For this review, take the finished solid that the model builds, in its own axes (mm). Face numbers are marked on the shaded views. A direction names the side the tool comes from. Give positions to 0.01 mm unless a question says otherwise; leave off trailing zeros. Order: outer loops, then holes, each group sorted by start corner. A loop starts at its lowest first (then second) coordinate and runs counter-clockwise, first axis right, second up. Notation, with made-up numbers: (-7.75, 88) - (12.25, 88) arc R8 cw to (12.25, 98) - close; hole circle Ø5 at (44.5, -34). An arc over 180 degrees is marked (long way). Use a Markdown table: item, result. Add a question column.
1) Wall thickness on L1, parallel to Y at x = -84, z = -15; L2, parallel to Z at x = 92, y = 3: over which ranges is each line inside the solid? List them lowest first.
2) We need section B-B on z = -22. Write out the cut boundary in (x, y).
3) Machinability: for the marked faces 1 and 2, which of the approach directions +Z, -Z, +X, -X, +Y, -Y give a long, thin tool a straight path to every point of the face, cutting with its end or side? Answer none if there is none.
4) We need section C-C on y = 11. Write out the cut boundary in (x, z), then the cut area to 3 significant figures.
5) We need section A-A on x = -72.5. Write out the cut boundary in (y, z).
6) Clearance check with flat-ended pins moving along their axes: P1, Ø0.6, axis at x = -31, y = -19, coming from the -Z side; P2, Ø1.5, axis at x = 60.5, z = -20.5, coming from the +Y side; P3, Ø1, axis at y = -19.5, z = -17.5, coming from the +X side. State where each tip first meets the part, or that it passes through.
7) We need section D-D on x = 117. Write out the cut boundary in (y, z).
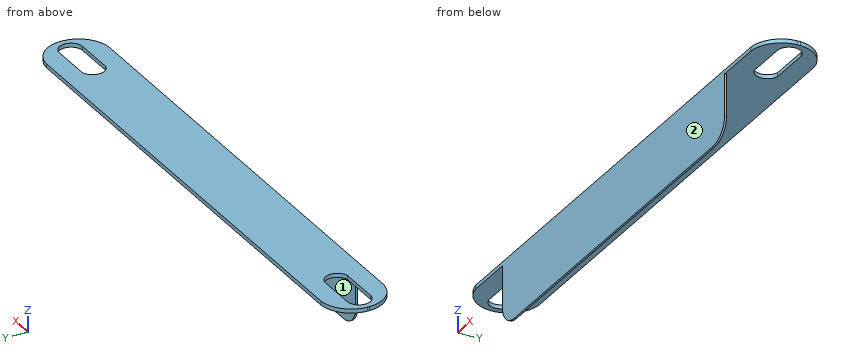
```python
from build123d import *

# Parameters (mm, degrees)
SKETCH1_W           = 351.028
SKETCH1_H           = 39.878
BOSS_EXTRUDE1_DEPTH = 2.54
CUT_EXTRUDE1_DEPTH  = 2.54
BOSS_EXTRUDE3_DEPTH = 1.27
CUT_EXTRUDE2_DEPTH  = 182.08885497


with BuildPart() as part:
    # Sketch1 → Boss-Extrude1 (new body)
    with BuildSketch(Plane.XY):
        Rectangle(SKETCH1_W, SKETCH1_H)
    extrude(amount=BOSS_EXTRUDE1_DEPTH)

    # Sketch2 → Cut-Extrude1 (cut)
    with BuildSketch(Plane.XY.offset(2.54)):
        with BuildLine():
            ThreePointArc((-175.514, 0.560558273), (-169.838630059, 13.933642373), (-156.610444921, 19.939))
            Line((-156.610444921, 19.939), (-175.514, 19.939))
            Line((-175.514, 19.939), (-175.514, 0.560558273))
        make_face()
        with BuildLine():
            ThreePointArc((-157.487509507, -19.939), (-170.14228569, -13.682666917), (-175.514, -0.627792376))
            Line((-175.514, -0.627792376), (-175.514, -19.939))
            Line((-175.514, -19.939), (-157.487509507, -19.939))
        make_face()
        with BuildLine():
            Line((175.514, 19.939), (156.589507007, 19.939))
            ThreePointArc((156.589507007, 19.939), (169.681715457, 14.129412549), (175.514, 1.047299362))
            Line((175.514, 1.047299362), (175.514, 19.939))
        make_face()
        with BuildLine():
            Line((175.514, -19.939), (175.514, -1.047299362))
            ThreePointArc((175.514, -1.047299362), (169.681715457, -14.129412549), (156.589507007, -19.939))
            Line((156.589507007, -19.939), (175.514, -19.939))
        make_face()
    extrude(amount=-CUT_EXTRUDE1_DEPTH, mode=Mode.SUBTRACT)

    # Sketch4 → Boss-Extrude3 (add)
    with BuildSketch(Plane(origin=(0, -19.939, 0), x_dir=(-1, 0, 0), z_dir=(0, -1, 0))):
        with BuildLine():
            Line((-126.490507007, 27.129664964), (-126.490507007, 0))
            Line((-126.490507007, 0), (127.388509507, 0))
            Line((127.388509507, 0), (127.388509507, 26.231634315))
            ThreePointArc((127.388509507, 26.231634315), (123.395271006, 35.875988979), (113.754553273, 39.878))
            Line((113.754553273, 39.878), (-112.615934561, 39.878))
            ThreePointArc((-112.615934561, 39.878), (-122.105920459, 36.282047556), (-126.490507007, 27.129664964))
        make_face()
    extrude(amount=-BOSS_EXTRUDE3_DEPTH)

    # Sketch5 → Cut-Extrude2 (cut, through all)
    with BuildSketch(Plane(origin=(0, 0, 0), x_dir=(-1, 0, 0), z_dir=(0, 0, -1))):
        with BuildLine():
            Line((-164.606102616, 7.415708173), (-138.164214663, 7.415708173))
            ThreePointArc((-138.164214663, 7.415708173), (-132.284701758, -0.002856694), (-138.164214663, -7.42142156))
            Line((-138.164214663, -7.42142156), (-164.606102616, -7.42142156))
            ThreePointArc((-164.606102616, -7.42142156), (-171.773613025, -0.002856694), (-164.606102616, 7.415708173))
        make_face()
    cut_extrude2 = extrude(amount=-CUT_EXTRUDE2_DEPTH, mode=Mode.SUBTRACT)

    # Mirror1: Cut-Extrude2 across plane
    add(cut_extrude2.mirror(Plane(origin=(0, 0, 0), x_dir=(0, 0, 1), z_dir=(1, 0, 0))), mode=Mode.SUBTRACT)


solid = part.part
```
Checked values:
| question | item | result |
|---|---|---|
| 1 | L1 | -19.94 to -18.67 |
| 1 | L2 | 0 to 2.54 |
| 2 | outline | (-127.39, -19.94) - (126.49, -19.94) - (126.49, -18.67) - (-127.39, -18.67) - close |
| 3 | face 1 | -Z, +X, -X, +Y |
| 3 | face 2 | +Z, -Z, +X, -X, -Y |
| 4 | outline | (-172.2, 0) - (172.24, 0) - (172.24, 2.54) - (-172.2, 2.54) - close |
| 4 | area | 875 mm² |
| 5 | outline | (-19.94, -39.88) - (-18.67, -39.88) - (-18.67, 0) - (19.94, 0) - (19.94, 2.54) - (-19.94, 2.54) - close |
| 6 | P1 | z = -39.88 |
| 6 | P2 | y = -18.67 |
| 6 | P3 | x = 126.49 |
| 7 | outline | (-19.94, -39.24) - (-18.67, -39.24) - (-18.67, 0) - (19.94, 0) - (19.94, 2.54) - (-19.94, 2.54) - close |
